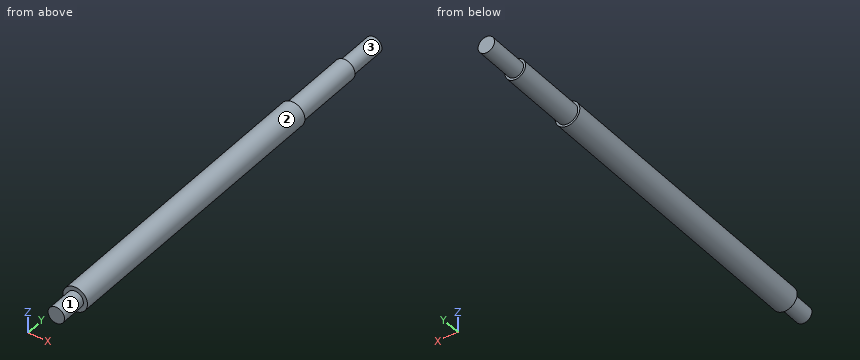
from build123d import *

# Parameters (mm, degrees)
F0_R     = 6
F1_DEPTH = 150
F2_R     = 5
F3_DEPTH = 36
F4_R     = 4
F5_DEPTH = 20
F6_R     = 4
F7_DEPTH = 13


with BuildPart() as f1:
    # F0 (on Front) → F1 (new body)
    with BuildSketch(Plane.XZ):
        Circle(F0_R)
    extrude(amount=F1_DEPTH)

    # F2 (on face) → F3 (join)
    with BuildSketch(Plane(origin=(0, 0, 0), x_dir=(-1, 0, 0), z_dir=(0, 1, 0))):
        Circle(F2_R)
    extrude(amount=F3_DEPTH)

    # F4 (on face) → F5 (join)
    with BuildSketch(Plane(origin=(0, 36, 0), x_dir=(-1, 0, 0), z_dir=(0, 1, 0))):
        Circle(F4_R)
    extrude(amount=F5_DEPTH)

    # F6 (on face) → F7 (join)
    with BuildSketch(Plane.XZ.offset(150)):
        Circle(F6_R)
    extrude(amount=F7_DEPTH)


solid = f1.part
Work out the finished part from the listing and answer in its coordinate system (mm). Face numbers are marked on the shaded views. A direction names the side the tool comes from. Round coordinates to 2 decimals unless told otherwise and drop trailing zeros. Write each loop counter-clockwise with the first axis right and the second up, starting at its lowest first coordinate (ties: lowest second). Pieces come first, ordered by that corner, then holes. Notation, with made-up numbers: (32.5, 56.5) -> (67.5, 56.5) arc R29 ccw to (67.5, 79.5) -> close; hole circle Ø7 at (50.5, -32.75). An arc over 180 degrees is marked (long way). Answer as CSV lines item,"result". Start each with the question number.
(1) The part is cut by section B-B, the plane x = 0. Give the vertices of the cut face in (y, z).
(2) The part is cut by section C-C, the plane y = 18. Give the vertices of the cut face in (x, z), then the cut area to 3 significant figures.
(3) The part is cut by section D-D, the plane y = -112. Give the vertices of the cut face in (x, z).
(4) The part is cut by section A-A, the plane z = 0. Give the vertices of the cut face in (x, y).
(5) Find the intervals of material crossed by probe 1 along Z at (x, y) = (0.5, 24.5); probe 2 along Z at (x, y) = (4.5, -1); probe 3 along Y at (x, z) = (-1, -4.25), in increasing order.
(6) A tool of negligible diameter and unlimited length cuts with its end or side. For the marked faces 1, 2 and 3, from which of +Z, -Z, +X, -X, +Y, -Y can it reach the whole face along a straight path? Write none if from no direction.
(7) Each of these flat-tipped pins is pushed along its axis until it touches: pin 1 (1 mm diameter, centred on y = 17, z = 4.5, fed in from +X); pin 2 (1.5 mm diameter, centred on x = -2, y = -11.5, fed in from -Z); pin 3 (1.5 mm diameter, centred on y = 17.5, z = -1.5, fed in from +X). Where does it stop, or does it pass through?
Output values:
1,outline,"(-163, -4) -> (-150, -4) -> (-150, -6) -> (0, -6) -> (0, -5) -> (36, -5) -> (36, -4) -> (56, -4) -> (56, 4) -> (36, 4) -> (36, 5) -> (0, 5) -> (0, 6) -> (-150, 6) -> (-150, 4) -> (-163, 4) -> close"
2,outline,"circle Ø10 at (0, 0)"
2,area,"78.5 mm²"
3,outline,"circle Ø12 at (0, 0)"
4,outline,"(-6, -150) -> (-4, -150) -> (-4, -163) -> (4, -163) -> (4, -150) -> (6, -150) -> (6, 0) -> (5, 0) -> (5, 36) -> (4, 36) -> (4, 56) -> (-4, 56) -> (-4, 36) -> (-5, 36) -> (-5, 0) -> (-6, 0) -> close"
5,probe 1,"z = -4.97 to 4.97"
5,probe 2,"z = -3.97 to 3.97"
5,probe 3,"y = -150 to 36"
6,face 1,"-Y"
6,face 2,"+Y, -Y"
6,face 3,"+Y"
7,pin 1,"stops at x = 3"
7,pin 2,"stops at z = -5.87"
7,pin 3,"stops at x = 4.94"
